Work out the finished part from the listing and answer in its coordinate system (mm). A direction names the side the tool comes from. Coordinates: 2 decimals unless noted, no trailing zeros. Loops run counter-clockwise (first coordinate to the right, second up) from the corner with the lowest first, then second, coordinate; pieces in that order, holes last. Notation, with made-up numbers: (55, 2) -> (78, 2) arc R22 cw to (78, 31) -> close; hole circle Ø11 at (71, 31). An arc over 180 degrees is marked (long way). Answer as CSV lines item,"result".
```python
from build123d import *

# Parameters (mm, degrees)
SKETCH_1_W          = 200
SKETCH_1_H          = 191
SKETCH_1_R          = 40
SKETCH_1_R_2        = 7.35
EXTRUDE_1_DEPTH     = 9
SKETCH_2_R          = 52
SKETCH_2_R_2        = 40
EXTRUDE_2_DEPTH     = 9
SKETCH_3_R          = 1.55
CUT_EXTRUDE_1_DEPTH = 9


with BuildPart() as part:
    # 草图1 → 凸台-拉伸1 (new body)
    with BuildSketch(Plane.XY):
        Rectangle(SKETCH_1_W, SKETCH_1_H)
        with Locations((0, -4.5)):
            Circle(SKETCH_1_R, mode=Mode.SUBTRACT)
        with Locations((-79.057591623, -75.5)):
            Circle(SKETCH_1_R_2, mode=Mode.SUBTRACT)
        with Locations((79.057591623, -75.5)):
            Circle(SKETCH_1_R_2, mode=Mode.SUBTRACT)
    extrude(amount=EXTRUDE_1_DEPTH)

    # 草图2 → 凸台-拉伸2 (add)
    with BuildSketch(Plane.XY.offset(9)):
        with Locations((0, -4.5)):
            Circle(SKETCH_2_R)
        with Locations((0, -4.5)):
            Circle(SKETCH_2_R_2, mode=Mode.SUBTRACT)
    extrude(amount=EXTRUDE_2_DEPTH)

    # 草图3 → 切除-拉伸1 (cut)
    with BuildSketch(Plane.XY.offset(18)):
        with Locations((1e-09, 41.5)):
            Circle(SKETCH_3_R)
        with Locations((39.837168574, 18.5)):
            Circle(SKETCH_3_R)
        with Locations((39.837168574, -27.5)):
            Circle(SKETCH_3_R)
        with Locations((0, -50.5)):
            Circle(SKETCH_3_R)
        with Locations((-39.837168574, -27.5)):
            Circle(SKETCH_3_R)
        with Locations((-39.837168574, 18.5)):
            Circle(SKETCH_3_R)
    extrude(amount=-CUT_EXTRUDE_1_DEPTH, mode=Mode.SUBTRACT)


solid = part.part
```
(1) Which of the six approach directions +Z, -Z, +X, -X, +Y, -Y give full straight-line access (tool end or side, diameter ignored) to faces 5 (the face through (-1, 95.5, 4)), 6 (the face through (-24, 44, 9))?
Computed values:
face 5,"+Z, -Z, +X, -X, +Y"
face 6,"+Z"
(2) A cutting plane is placed at B-B, the plane y = -75.5. Write down the section's boundary in (x, z).
Computed values:
outline,"(-100, 0) -> (-86.41, 0) -> (-86.41, 9) -> (-100, 9) -> close; (-71.71, 0) -> (71.71, 0) -> (71.71, 9) -> (-71.71, 9) -> close; (86.41, 0) -> (100, 0) -> (100, 9) -> (86.41, 9) -> close"
(3) For a pull along X with two mould halves and no side action, classify faces 1 (the face through (11.3, 34.3, 18)), 2 (the face through (71.715, -75.177, 4.437)), 3 (the face through (-41.265, -36.141, 13.437)), 4 (the face through (-86.4, -75.2, 4.4)) as pulls with the +X half, pulls with the -X half, needs draft (parallel to the pull), parting line crosses it, or undercut.
Computed values:
face 1,"needs draft"
face 2,"undercut"
face 3,"parting line crosses it"
face 4,"undercut"
(4) A cutting plane is placed at C-C, the plane z = 14. Write down the section's boundary in (x, y), and give its area (3 significant figures).
Computed values:
outline,"circle Ø104 at (0, -4.5); hole circle Ø3.1 at (-39.84, -27.5); hole circle Ø3.1 at (-39.84, 18.5); hole circle Ø80 at (0, -4.5); hole circle Ø3.1 at (0, -50.5); hole circle Ø3.1 at (0, 41.5); hole circle Ø3.1 at (39.84, -27.5); hole circle Ø3.1 at (39.84, 18.5)"
area,"3,420 mm2"
(5) A cutting plane is placed at A-A, the plane y = -4.5. Write down the section's boundary in (x, z).
Computed values:
outline,"(-100, 0) -> (-40, 0) -> (-40, 18) -> (-52, 18) -> (-52, 9) -> (-100, 9) -> close; (40, 0) -> (100, 0) -> (100, 9) -> (52, 9) -> (52, 18) -> (40, 18) -> close"
(6) A cutting plane is placed at D-D, the plane x = -44. Write down the section's boundary in (y, z), and give its area (3 significant figures).
Computed values:
outline,"(-95.5, 0) -> (95.5, 0) -> (95.5, 9) -> (23.21, 9) -> (23.21, 18) -> (-32.21, 18) -> (-32.21, 9) -> (-95.5, 9) -> close"
area,"2,220 mm2"
(7) Flat-ended cylindrical pins translate along their axes: pin 1 Ø2.5 at (x, y) = (0, 41.5) entering from -Z; pin 2 Ø3 at (x, y) = (-64.5, -21) entering from +Z; pin 3 Ø1 at (y, z) = (-37.5, 15) entering from -X. Find the tip coordinate at first contact, or state that the pin passes through.
Computed values:
pin 1,"z = 0"
pin 2,"z = 9"
pin 3,"x = -40.59"
(8) Consider line 1 along Y through (x, z) = (0, 11.75); line 2 along Y through (x, z) = (0, 7.75); line 3 along Z through (x, y) = (-59.5, -78). Determine where each line is inside the solid, lowest interval first.
Computed values:
line 1,"-56.5 to -52.05, -48.95 to -44.5, 35.5 to 39.95, 43.05 to 47.5"
line 2,"-95.5 to -44.5, 35.5 to 95.5"
line 3,"0 to 9"
